Study the drawing (mm; zero at the part's minimum x, y, z) and answer. Coordinates: 2 decimals unless noted, no trailing zeros. Write each loop counter-clockwise with the first axis right and the second up, starting at its lowest first coordinate (ties: lowest second). Pieces come first, ordered by that corner, then holes. Notation, with made-up numbers: (-12.5, -17.5) -> (13.5, -17.5) arc R37 ccw to (13.5, 20.5) -> close; hole circle Ø2 at (77.25, 59). An arc over 180 degrees is marked (long way). Write item = value, one per line. Start each with the question number.
1) Section C-C (y = 26) is taken. Determine the outline of the cut face in (x, z), plus the area to 3 significant figures.
2) Section B-B (x = 100) is taken. Determine the outline of the cut face in (y, z).
3) A flat-ended cylindrical pin translates along its axis: pin 1 Ø1 at (x, z) = (122, 1.5) entering from +Y. Find the tip coordinate at first contact, or state that the pin passes through.
4) Find the intervals of material crossed by line 1 along Y through (x, z) = (100, 1.05); line 2 along X through (y, z) = (70.5, 1.9); line 3 along X through (y, z) = (58, 1.3), in increasing order. Write a range as from..to.
5) Section A-A (y = 50) is taken. Determine the outline of the cut face in (x, z), plus the area to 3 significant figures.
6) Section D-D (x = 72) is taken. Determine the outline of the cut face in (y, z).
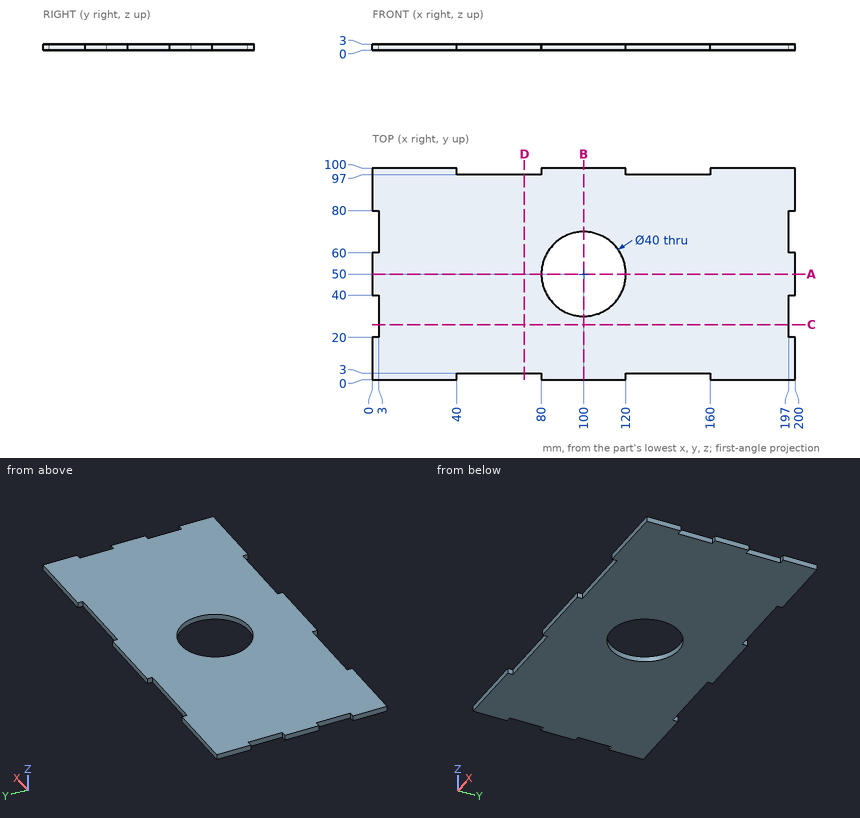
Answer key:
q1.outline = (3, 0) -> (197, 0) -> (197, 3) -> (3, 3) -> close
q1.area = 582 mm^2
q2.outline = (0, 0) -> (30, 0) -> (30, 3) -> (0, 3) -> close; (70, 0) -> (100, 0) -> (100, 3) -> (70, 3) -> close
q3.pin_1 = 97
q4.line_1 = 0..30, 70..100
q4.line_2 = 3..197
q4.line_3 = 0..81.67, 118.33..200
q5.outline = (0, 0) -> (80, 0) -> (80, 3) -> (0, 3) -> close; (120, 0) -> (200, 0) -> (200, 3) -> (120, 3) -> close
q5.area = 480 mm^2
q6.outline = (3, 0) -> (97, 0) -> (97, 3) -> (3, 3) -> close
